```python
from build123d import *

# Parameters (mm, degrees)
F0_W     = 62.077142
F0_H     = 59.255235
F1_DEPTH = 14.824914
F2_W     = 70.476621
F2_H     = 59.255235
F3_DEPTH = 25.4
F4_W     = 10.496232
F4_H     = 45.620956
F5_DEPTH = 83.277501
F6_R     = 5.256792
F7_DEPTH = 12.7
F9_D     = 6.35


with BuildPart() as f1:
    # F0 (on Front) → F1 (new body)
    with BuildSketch(Plane.XZ):
        with Locations((31.038571, 29.627617)):
            Rectangle(F0_W, F0_H)
    extrude(amount=-F1_DEPTH)

    # F2 (on face) → F3 (join)
    with BuildSketch(Plane.YZ.offset(62.077142)):
        with Locations((35.23831, 29.627617)):
            Rectangle(F2_W, F2_H)
    extrude(amount=F3_DEPTH)

    # F4 (on face) → F5 (join)
    with BuildSketch(Plane.YZ.offset(87.477142)):
        with Locations((65.228505, 22.810478)):
            Rectangle(F4_W, F4_H)
    extrude(amount=F5_DEPTH)

    # F6 (on face) → F7 (join, symmetric)
    with BuildSketch(Plane(origin=(0, 70.476621, 0), x_dir=(-1, 0, 0), z_dir=(0, 1, 0))):
        with Locations((-137.36628, 24.403818)):
            Circle(F6_R)
    extrude(amount=F7_DEPTH, both=True)

    # F9 (through all)
    with Locations(Plane.YZ.offset(87.477142)):
        with Locations((16.669355, 23.290077), (36.526144, 32.229573), (38.65239, 52.261315)):
            Hole(F9_D / 2)


solid = f1.part
```
Verification items for the finished model (mm, model axes). A direction names the side the tool comes from. Round coordinates to 2 decimals unless told otherwise and drop trailing zeros. Write each loop counter-clockwise with the first axis right and the second up, starting at its lowest first coordinate (ties: lowest second). Pieces come first, ordered by that corner, then holes. Notation, with made-up numbers: (0.5, 82.25) -> (26.5, 82.25) arc R21 cw to (26.5, 114.25) -> close; hole circle Ø3 at (48.25, 11). An arc over 180 degrees is marked (long way). Write each question's results on one line, items separated by ' | '.
Q1. Draft check along Z on faces 4 (the face through (31, 14.825, 43)), 5 (the face through (63, 27, 0)), 6 (the face through (62.57, 13.64, 24.24)). Enter one of: released by +Z, released by -Z, zero draft, split by the parting line, or undercut.
Derived:
face 4: zero draft | face 5: released by -Z | face 6: undercut
Q2. Sectioned sample at D-D, the plane x = 139. Record the boundary of the cut face in (y, z).
Derived:
outline: (57.78, 19.41) -> (59.98, 19.41) -> (59.98, 0) -> (70.48, 0) -> (70.48, 19.41) -> (83.18, 19.41) -> (83.18, 29.4) -> (70.48, 29.4) -> (70.48, 45.62) -> (59.98, 45.62) -> (59.98, 29.4) -> (57.78, 29.4) -> close
Q3. Sectioned sample at C-C, the plane x = 75. Record the boundary of the cut face in (y, z) (3 decimals), and give its area (3 significant figures).
Derived:
outline: (0, 0) -> (70.477, 0) -> (70.477, 59.255) -> (0, 59.255) -> close; hole circle Ø6.35 at (16.669, 23.29); hole circle Ø6.35 at (36.526, 32.23); hole circle Ø6.35 at (38.652, 52.261) | area: 4,080 mm²
Q4. Sectioned sample at B-B, the plane z = 43. Record the boundary of the cut face in (x, y).
Derived:
outline: (0, 0) -> (87.48, 0) -> (87.48, 59.98) -> (170.75, 59.98) -> (170.75, 70.48) -> (62.08, 70.48) -> (62.08, 14.82) -> (0, 14.82) -> close
Q5. Thickness scan on probe 1 along X at (y, z) = (31, 35); probe 2 along Y at (x, z) = (103, 34.5); probe 3 along Y at (x, z) = (25.5, 13.5). Record the ranges inside material, lowest first.
Derived:
probe 1: x = 62.08 to 87.48 | probe 2: y = 59.98 to 70.48 | probe 3: y = 0 to 14.82
Q6. Access from +Z, -Z, +X, -X, +Y, -Y to the whole of each face (thin tool, end or side, straight path). Record for faces 1 (the face through (75, 70.477, 29)), 2 (the face through (142.62, 58.89, 24.63)), 3 (the face through (142.62, 76.92, 24.63)).
Derived:
face 1: +Z, -Z, -X, +Y | face 2: -Y | face 3: +Y
Q7. Sectioned sample at A-A, the plane y = 64. Record the boundary of the cut face in (x, z), and give its area (3 significant figures).
Derived:
outline: (62.08, 0) -> (170.75, 0) -> (170.75, 45.62) -> (87.48, 45.62) -> (87.48, 59.26) -> (62.08, 59.26) -> close | area: 5,300 mm²
Q8. Go/stop test with flat-tipped pins: pin 1 Ø11.5 at (x, z) = (134.5, 26) entering from -Y; pin 2 Ø10 at (y, z) = (50, 35.5) entering from +X; pin 3 Ø16.5 at (y, z) = (33.5, 22.5) entering from -X. Record where each tip stops, or that it passes through.
Derived:
pin 1: stops at y = 57.78 | pin 2: stops at x = 87.48 | pin 3: stops at x = 62.08
